from build123d import *

# Parameters (mm, degrees)
SKETCH1_W            = 63.8
SKETCH1_H            = 73.8
SKETCH1_R            = 28.25
BOSS_EXTRUDE19_DEPTH = 10
SKETCH1_16_W         = 63.8
SKETCH1_16_H         = 73.8
SKETCH1_16_R         = 28.25
BOSS_EXTRUDE20_DEPTH = 50
CUT_EXTRUDE1_DEPTH   = 100


with BuildPart() as part:
    # Sketch1 → Boss-Extrude19 (new body)
    with BuildSketch(Plane.XY):
        Rectangle(SKETCH1_W, SKETCH1_H)
        Circle(SKETCH1_R, mode=Mode.SUBTRACT)
        with BuildLine():
            Line((-26.694444444, -16.722937415), (-26.694444444, -31))
            Line((-26.694444444, -31), (-5.590169944, -31))
            ThreePointArc((-5.590169944, -31), (-17.650289249, -26.090559393), (-26.694444444, -16.722937415))
        make_face(mode=Mode.SUBTRACT)
        with BuildLine():
            Line((5.590169944, -31), (26.694444444, -31))
            Line((26.694444444, -31), (26.694444444, -16.722937415))
            ThreePointArc((26.694444444, -16.722937415), (17.650289249, -26.090559393), (5.590169944, -31))
        make_face(mode=Mode.SUBTRACT)
        with BuildLine():
            Line((5.590169944, 31), (26.694444444, 31))
            Line((26.694444444, 31), (26.694444444, 16.722937415))
            ThreePointArc((26.694444444, 16.722937415), (17.650289249, 26.090559393), (5.590169944, 31))
        make_face(mode=Mode.SUBTRACT)
        with BuildLine():
            Line((-26.694444444, 31), (-5.590169944, 31))
            ThreePointArc((-5.590169944, 31), (-17.650289249, 26.090559393), (-26.694444444, 16.722937415))
            Line((-26.694444444, 16.722937415), (-26.694444444, 31))
        make_face(mode=Mode.SUBTRACT)
    extrude(amount=BOSS_EXTRUDE19_DEPTH)

    # Sketch1_16 → Boss-Extrude20 (add)
    with BuildSketch(Plane.XY):
        Rectangle(SKETCH1_16_W, SKETCH1_16_H)
        Circle(SKETCH1_16_R, mode=Mode.SUBTRACT)
        with BuildLine():
            Line((-26.694444444, -16.722937415), (-26.694444444, -31))
            Line((-26.694444444, -31), (-5.590169944, -31))
            ThreePointArc((-5.590169944, -31), (-17.650289249, -26.090559393), (-26.694444444, -16.722937415))
        make_face(mode=Mode.SUBTRACT)
        with BuildLine():
            Line((5.590169944, -31), (26.694444444, -31))
            Line((26.694444444, -31), (26.694444444, -16.722937415))
            ThreePointArc((26.694444444, -16.722937415), (17.650289249, -26.090559393), (5.590169944, -31))
        make_face(mode=Mode.SUBTRACT)
        with BuildLine():
            Line((5.590169944, 31), (26.694444444, 31))
            Line((26.694444444, 31), (26.694444444, 16.722937415))
            ThreePointArc((26.694444444, 16.722937415), (17.650289249, 26.090559393), (5.590169944, 31))
        make_face(mode=Mode.SUBTRACT)
        with BuildLine():
            Line((-26.694444444, 31), (-5.590169944, 31))
            ThreePointArc((-5.590169944, 31), (-17.650289249, 26.090559393), (-26.694444444, 16.722937415))
            Line((-26.694444444, 16.722937415), (-26.694444444, 31))
        make_face(mode=Mode.SUBTRACT)
    extrude(amount=BOSS_EXTRUDE20_DEPTH)

    # Sketch7 → Cut-Extrude1 (cut)
    with BuildSketch(Plane(origin=(40, 0, 0), x_dir=(0, 0, -1), z_dir=(1, 0, 0))):
        with BuildLine():
            Line((-42, 2.1), (-8, 2.1))
            ThreePointArc((-8, 2.1), (-5.9, 0), (-8, -2.1))
            Line((-8, -2.1), (-42, -2.1))
            ThreePointArc((-42, -2.1), (-44.1, 0), (-42, 2.1))
        make_face()
    extrude(amount=-CUT_EXTRUDE1_DEPTH, mode=Mode.SUBTRACT)


solid = part.part
Here's how the part is built. I have some questions about the finished solid (model axes, mm). A direction names the side the tool comes from. Give positions to 0.01 mm unless a question says otherwise; leave off trailing zeros. Loops run counter-clockwise (first coordinate to the right, second up) from the corner with the lowest first, then second, coordinate; pieces in that order, holes last. Notation, with made-up numbers: (64, 86) -> (111, 86) arc R21 ccw to (111, 96) -> close; hole circle Ø8 at (25.5, 31). An arc over 180 degrees is marked (long way). Answer as a JSON object with one key per item and string values. Group by question number.
Item 1: Imagine slicing it at D-D on x = -25. Write out the boundary of the cut face in (y, z).
Item 2: Thinking about a two-plate mould opening in Y: for faces 1 (the flat face through (-30, 2.1, 25)), 2 (the flat face through (-15, 25, 0)), 3 (the flat face through (0, 36.9, 25)), which applies, pulls with the +Y half, pulls with the -Y half, needs draft (parallel to the pull), parting line crosses it, or undercut?
Item 3: Imagine slicing it at A-A on z = 25.5. Write out the boundary of the cut face in (x, y).
Item 4: Imagine slicing it at B-B on x = 0. Write out the boundary of the cut face in (y, z), then the cut area to 3 significant figures.
Item 5: I need wall thicknesses on L1, parallel to Y at x = 0, z = 12; L2, parallel to Y at x = 11, z = 11; L3, parallel to X at y = 23, z = 38. Which ranges of each line are inside material? Lowest first, please.
Item 6: On a 3-axis mill with a long thin cutter (end or side, diameter ignored), from which of +Z, -Z, +X, -X, +Y, -Y can I reach the whole of each face in a straight line? I mean faces 4 (the flat face through (-26.694, -24, 25)), 5 (the flat face through (-15, 25, 50)), 6 (the cylindrical face through (-30, 0, 44.1)). Say none if no direction works.
Item 7: Imagine slicing it at C-C on y = 0. Write out the boundary of the cut face in (x, z), then the cut area to 3 significant figures.
Answer list:
{
 "1": {"outline": "(-36.9, 0) -> (-31, 0) -> (-31, 50) -> (-36.9, 50) -> close; (-19.16, 0) -> (-13.16, 0) -> (-13.16, 50) -> (-19.16, 50) -> close; (13.16, 0) -> (19.16, 0) -> (19.16, 50) -> (13.16, 50) -> close; (31, 0) -> (36.9, 0) -> (36.9, 50) -> (31, 50) -> close"},
 "2": {"face 1": "undercut", "face 2": "needs draft", "face 3": "pulls with the +Y half"},
 "3": {"outline": "(-31.9, -36.9) -> (31.9, -36.9) -> (31.9, -2.1) -> (28.17, -2.1) arc R28.25 cw to (-28.17, -2.1) -> (-31.9, -2.1) -> close; (-31.9, 2.1) -> (-28.17, 2.1) arc R28.25 cw to (28.17, 2.1) -> (31.9, 2.1) -> (31.9, 36.9) -> (-31.9, 36.9) -> close; hole (-26.69, -31) -> (-5.59, -31) arc R31.5 cw to (-26.69, -16.72) -> close; hole (-26.69, 16.72) arc R31.5 cw to (-5.59, 31) -> (-26.69, 31) -> close; hole (5.59, -31) -> (26.69, -31) -> (26.69, -16.72) arc R31.5 cw to start; hole (5.59, 31) arc R31.5 cw to (26.69, 16.72) -> (26.69, 31) -> close"},
 "4": {"outline": "(-36.9, 0) -> (-28.25, 0) -> (-28.25, 50) -> (-36.9, 50) -> close; (28.25, 0) -> (36.9, 0) -> (36.9, 50) -> (28.25, 50) -> close", "area": "865 mm2"},
 "5": {"L1": "y = -36.9 to -28.25, 28.25 to 36.9", "L2": "y = -36.9 to -31, -29.52 to -26.02, 26.02 to 29.52, 31 to 36.9", "L3": "x = -31.9 to -26.69, -21.52 to -16.4, 16.4 to 21.52, 26.69 to 31.9"},
 "6": {"face 4": "+Z, -Z", "face 5": "+Z, +X, -X, +Y, -Y", "face 6": "+X, -X"},
 "7": {"outline": "(-31.9, 0) -> (-28.25, 0) -> (-28.25, 5.9) -> (-31.9, 5.9) -> close; (-31.9, 44.1) -> (-28.25, 44.1) -> (-28.25, 50) -> (-31.9, 50) -> close; (28.25, 0) -> (31.9, 0) -> (31.9, 5.9) -> (28.25, 5.9) -> close; (28.25, 44.1) -> (31.9, 44.1) -> (31.9, 50) -> (28.25, 50) -> close", "area": "86.1 mm2"}
}
